Work out the finished part from the listing and answer in its coordinate system (mm). A direction names the side the tool comes from. Coordinates: 2 decimals unless noted, no trailing zeros. Answer as a JSON object with one key per item and string values. Group by question number.
1) Find the intervals of material crossed by line 1 along X through (y, z) = (-2.3, -3.9); line 2 along Y through (x, z) = (0, 0.75); line 3 along X through (y, z) = (2.15, -3.9), in increasing order.
2) Each of these flat-tipped pins is pushed along its axis until it touches: P1, Ø5, axis at y = 2, z = -4, coming from the -X side; P2, Ø2.5, axis at x = 0, z = -3.9, coming from the +Y side; P3, Ø6, axis at x = -4.5, y = 1, coming from the -Z side. Where does it stop, or does it pass through?
3) A tool of negligible diameter and unlimited length cuts with its end or side. For faces 4 (the face through (0, 2, 1)), 5 (the face through (3, 0, 7.6)), from which of +Z, -Z, +X, -X, +Y, -Y can it reach the whole face along a straight path? Write none if from no direction.
4) The mould has two halves that part along Z. Classify faces 1 (the face through (-0.216, -2.44, -2.926)), 2 (the face through (-4.8, 2, 4.3)), 3 (the face through (0, 0, -5.9)): released by +Z, released by -Z, zero draft, split by the parting line, or undercut.
from build123d import *

# Parameters (mm, degrees)
CROQUIS2_R            = 0.99756867
CORTAR_EXTRUIR1_DEPTH = 5
CROQUIS4_R            = 2
CORTAR_EXTRUIR2_DEPTH = 13.5
CHAFL_N1_SIZE         = 0.5


with BuildPart() as part:
    # Croquis1 → Revolución1 (revolve)
    with BuildSketch(Plane(origin=(0, 0, 0), x_dir=(1, 0, 0), z_dir=(0, 1, 0))):
        with BuildLine():
            Line((0, -7.6), (-6.5, -7.6))
            Line((-6.5, -7.6), (-6.5, -5.6))
            Line((-6.5, -5.6), (-5.085786438, -4.185786438))
            add(Edge.make_bspline(
                [(-5.085786438, -4.185786438), (-4.45743914, 2.686299208), (-1.971742684, 7.41138075), (0, 7.6)],
                knots=[0, 0, 0, 0, 1, 1, 1, 1], degree=3))
            Line((0, 7.6), (0, -7.6))
        make_face()
    revolve(axis=Axis((0, 0, -14.344827586), (0, 0, 1)))

    # Croquis2 → Cortar-Extruir1 (cut, symmetric)
    with BuildSketch(Plane(origin=(0, 0, 0), x_dir=(1, 0, 0), z_dir=(0, 1, 0))):
        with Locations((0, 3.9)):
            Circle(CROQUIS2_R)
    extrude(amount=CORTAR_EXTRUIR1_DEPTH, both=True, mode=Mode.SUBTRACT)

    # Croquis4 → Cortar-Extruir2 (cut)
    with BuildSketch(Plane.XY.offset(7.6)):
        Circle(CROQUIS4_R)
    extrude(amount=-CORTAR_EXTRUIR2_DEPTH, mode=Mode.SUBTRACT)

    # Chaflán1
    chafl_n1_edges = [part.edges().sort_by_distance(p)[0] for p in [
        (-2, 0, 7.6),
    ]]
    chamfer(chafl_n1_edges, length=CHAFL_N1_SIZE)


solid = part.part
Report:
{
 "1": {"line 1": "x = -2.21 to -1, 1 to 2.21", "line 2": "y = -4.59 to -2, 2 to 4.59", "line 3": "x = -2.35 to -1, 1 to 2.35"},
 "2": {"P1": "stops at x = -3.87", "P2": "stops at y = 3.67", "P3": "stops at z = -6.56"},
 "3": {"face 4": "+Z", "face 5": "+Z, +X, -X, +Y, -Y"},
 "4": {"face 1": "undercut", "face 2": "released by -Z", "face 3": "released by +Z"}
}
